Verification items for the finished model (mm, model axes). A direction names the side the tool comes from. Coordinates: 2 decimals unless noted, no trailing zeros. Write each loop counter-clockwise with the first axis right and the second up, starting at its lowest first coordinate (ties: lowest second). Pieces come first, ordered by that corner, then holes. Notation, with made-up numbers: M 79,33 L 96,33 A31 ccw 96,69 Z; hole C 57,49 d3. An arc over 180 degrees is marked long. One line per item, written item: value.
```python
from build123d import *

# Parameters (mm, degrees)
F1_DEPTH = 60
F2_R     = 3
F3_DEPTH = 8
F4_R     = 3
F5_DEPTH = 8


# Not quite as in the source:
# - a feature names something its author has since deleted; it is built from what else it names


with BuildPart() as f1:
    # F0 (on Front) → F1 (new body)
    with BuildSketch(Plane.XZ):
        Polygon((29.4997055829, 0), (6.2059915236, 86.933324366), (-40.5002944171, 86.933324366), (-40.5002944171, -10), (29.4997055829, -10), align=None)
    extrude(amount=F1_DEPTH)

    # F2 (on face) → F3 (cut)
    with BuildSketch(Plane(origin=(0, 0, -10), x_dir=(1, 0, 0), z_dir=(0, 0, -1))):
        with Locations((-30.5002944171, 30)):
            Circle(F2_R)
        with Locations((19.4997055829, 30)):
            Circle(F2_R)
    extrude(amount=-F3_DEPTH, mode=Mode.SUBTRACT)

    # F4 (on face) → F5 (cut)
    with BuildSketch(Plane(origin=(27.5236000109, 0, 7.3749263957), x_dir=(0, 1, 0), z_dir=(0.9659258263, 0, 0.2588190451))):
        with Locations((-30, 72.3649143702)):
            Circle(F4_R)
        with Locations((-30, 2.3649143702)):
            Circle(F4_R)
    extrude(amount=-F5_DEPTH, mode=Mode.SUBTRACT)


solid = f1.part
```
Item 1: Draft check along Z on faces 1 (the face through (19.173, -30.042, 7.629)), 2 (the face through (4.95, -32.997, 76.381)), 3 (the face through (-6, -30, -10)), 4 (the face through (-40.5, -30, 39)). Enter one of: released by +Z, released by -Z, zero draft, split by the parting line, or undercut.
The answers:
face 1: undercut
face 2: undercut
face 3: released by -Z
face 4: zero draft
Item 2: Scan lines: line 1 (X direction, y = -30, z = -4); line 2 (Z direction, x = 5.5, y = -29.5); line 3 (Z direction, x = 2, y = -31). Record each from-to range of solid material in increasing order.
The answers:
line 1: x = -40.5 to -33.5, -27.5 to 16.5, 22.5 to 29.5
line 2: z = -10 to 73.33, 79.45 to 86.93
line 3: z = -10 to 72.53, 78.38 to 86.93
Item 3: Access from +Z, -Z, +X, -X, +Y, -Y to the whole of each face (thin tool, end or side, straight path). Record for faces 5 (the face through (-31, -30, -2)), 6 (the face through (1.056, -30.042, 75.244)), 7 (the face through (18.016, -29.58, 42.858)).
The answers:
face 5: -Z
face 6: none
face 7: +Z, +X, +Y, -Y
Item 4: Cross-section at C-C, the plane x = 12. Enter the section's corners in (y, z), and give its area (3 significant figures).
The answers:
outline: M -60,-10 L 0,-10 L 0,65.31 L -60,65.31 Z
area: 4,520 mm²
Item 5: Cross-section at B-B, the plane z = 30.5. Enter the section's corners in (x, y).
The answers:
outline: M -40.5,-60 L 21.33,-60 L 21.33,0 L -40.5,0 Z
Item 6: Cross-section at A-A, the plane y = -34.5. Enter the section's corners in (x, z).
The answers:
outline: M -40.5,-10 L 29.5,-10 L 29.5,0 L 6.21,86.93 L -40.5,86.93 Z
Item 7: Go/stop test with flat-tipped pins: P1, Ø2, axis at y = -25, z = 31.5, coming from the +X side; P2, Ø3, axis at x = -30, y = -29, coming from the -Z side; P3, Ø12, axis at y = -10.5, z = 76, coming from the +X side. Record where each tip stops, or that it passes through.
The answers:
P1: stops at x = 21.33
P2: stops at z = -2
P3: stops at x = 10.74
